Could you check a few things on this model? Use its own coordinates, in mm. Face numbers are marked on the shaded views. A direction names the side the tool comes from. Round coordinates to 2 decimals unless told otherwise and drop trailing zeros. Loops run counter-clockwise (first coordinate to the right, second up) from the corner with the lowest first, then second, coordinate; pieces in that order, holes last. Notation, with made-up numbers: M 23.25,83.25 L 36.25,83.25 A32 cw 36.25,117.25 Z; hole C 87,76.5 d6. An arc over 180 degrees is marked long. Answer in a Markdown table with one row per item.
```python
from build123d import *

# Parameters (mm, degrees)
F1_DEPTH         = 16
F2_T             = -2.5
F3_R             = 1
F4_DEPTH         = 5.5
F4_COPIES2_COUNT = 2
F5_W             = 11.5
F5_H             = 11.5
F5_R             = 2.75
F6_DEPTH         = 2.501


# Not quite as in the source:
# - a pattern or mirror of a feature is missing from the dataset's text; its kind, count and spacing are read off the source's solid


with BuildPart() as f1:
    # F0 (on Top) → F1 (new body)
    with BuildSketch(Plane.XY):
        with BuildLine():
            ThreePointArc((36.12, 24.13), (33.9115851301, 29.4615851301), (28.58, 31.67))
            Line((28.58, 31.67), (-28.58, 31.67))
            ThreePointArc((-28.58, 31.67), (-33.9115851301, 29.4615851301), (-36.12, 24.13))
            Line((-36.12, 24.13), (-36.12, -24.13))
            ThreePointArc((-36.12, -24.13), (-33.9115851301, -29.4615851301), (-28.58, -31.67))
            Line((-28.58, -31.67), (28.58, -31.67))
            ThreePointArc((28.58, -31.67), (33.9115851301, -29.4615851301), (36.12, -24.13))
            Line((36.12, -24.13), (36.12, 24.13))
        make_face()
    extrude(amount=F1_DEPTH)

    # F2
    f2_openings = [f1.faces().sort_by_distance(p)[0] for p in [
        (0, 0, 16),
    ]]
    offset(amount=F2_T, openings=f2_openings)

    # F3 (on face) → F4 (join)
    with BuildSketch(Plane.XY.offset(2.5)):
        with BuildLine():
            Line((-26.04, 24.13), (-26.04, 29.17))
            Line((-26.04, 29.17), (-28.58, 29.17))
            ThreePointArc((-28.58, 29.17), (-32.1438181772, 27.6938181772), (-33.62, 24.13))
            Line((-33.62, 24.13), (-33.62, 21.59))
            Line((-33.62, 21.59), (-28.58, 21.59))
            ThreePointArc((-28.58, 21.59), (-26.7839487758, 22.3339487758), (-26.04, 24.13))
        make_face()
        with Locations((-28.58, 24.13)):
            Circle(F3_R, mode=Mode.SUBTRACT)
    f4 = extrude(amount=F4_DEPTH)

    # F4_copies: F4 across plane
    add(f4.mirror(Plane(origin=(0, 0, 0), x_dir=(0, 0, 1), z_dir=(1, 0, 0))))

    # F4_copies1: F4 across plane
    add(f4.mirror(Plane(origin=(0, 0, 0), x_dir=(0, 0, -1), z_dir=(0, -1, 0))))

    # F4_copies2: F4 ×2 about axis
    f4_copies2_axis = Axis((0, 0, 0), (0, 0, 1))
    for i in range(1, F4_COPIES2_COUNT):
        add(f4.rotate(f4_copies2_axis, i * 360 / F4_COPIES2_COUNT))

    # F5 (on face) → F6 (cut, through all)
    with BuildSketch(Plane.XY.offset(2.5)):
        with Locations((-18.42, 13.97)):
            Rectangle(F5_W, F5_H)
        with Locations((-5.72, 13.97)):
            Circle(F5_R)
        with Locations((-18.42, -6.35)):
            Rectangle(F5_W, F5_H)
        with Locations((-5.72, -6.35)):
            Circle(F5_R)
        with Locations((13.33, 13.97)):
            Rectangle(F5_W, F5_H)
        with Locations((26.03, 13.97)):
            Circle(F5_R)
        with Locations((13.33, -6.35)):
            Rectangle(F5_W, F5_H)
        with Locations((26.03, -6.35)):
            Circle(F5_R)
    extrude(amount=-F6_DEPTH, mode=Mode.SUBTRACT)


solid = f1.part
```
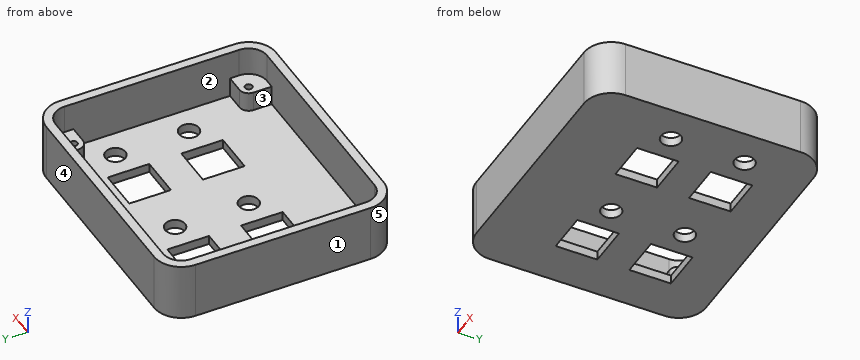
1) I want a section at C-C, the plane z = 5.5. Please give me the cut outline in (x, y).
Computed:
| item | result |
|---|---|
| outline | M -36.12,-24.13 A7.54 ccw -28.58,-31.67 L 28.58,-31.67 A7.54 ccw 36.12,-24.13 L 36.12,24.13 A7.54 ccw 28.58,31.67 L -28.58,31.67 A7.54 ccw -36.12,24.13 Z; hole M -33.62,-21.59 L -28.58,-21.59 A2.54 cw -26.04,-24.13 L -26.04,-29.17 L 26.04,-29.17 L 26.04,-24.13 A2.54 cw 28.58,-21.59 L 33.62,-21.59 L 33.62,21.59 L 28.58,21.59 A2.54 cw 26.04,24.13 L 26.04,29.17 L -26.04,29.17 L -26.04,24.13 A2.54 cw -28.58,21.59 L -33.62,21.59 Z; hole C -28.58,-24.13 d2; hole C -28.58,24.13 d2; hole C 28.58,-24.13 d2; hole C 28.58,24.13 d2 |
2) I want a section at D-D, the plane z = 10. Please give me the cut outline in (x, y), plus the area to 3 significant figures.
Computed:
| item | result |
|---|---|
| outline | M -36.12,-24.13 A7.54 ccw -28.58,-31.67 L 28.58,-31.67 A7.54 ccw 36.12,-24.13 L 36.12,24.13 A7.54 ccw 28.58,31.67 L -28.58,31.67 A7.54 ccw -36.12,24.13 Z; hole M -33.62,-24.13 A5.04 ccw -28.58,-29.17 L 28.58,-29.17 A5.04 ccw 33.62,-24.13 L 33.62,24.13 A5.04 ccw 28.58,29.17 L -28.58,29.17 A5.04 ccw -33.62,24.13 Z |
| area | 626 mm² |
3) I need wall thicknesses on line 1 (Y direction, x = 28.58, z = 5.25); line 2 (Y direction, x = -19, z = 5.25); line 3 (Y direction, x = 23.5, z = 1). Which ranges of each line are inside material? Lowest first, please.
Computed:
| item | result |
|---|---|
| line 1 | y = -31.67 to -25.13, -23.13 to -21.59, 21.59 to 23.13, 25.13 to 31.67 |
| line 2 | y = -31.67 to -29.17, 29.17 to 31.67 |
| line 3 | y = -31.67 to -7.43, -5.27 to 12.89, 15.05 to 31.67 |
4) I want a section at B-B, the plane y = -6.35. Please give me the cut outline in (x, z), plus the area to 3 significant figures.
Computed:
| item | result |
|---|---|
| outline | M -36.12,0 L -24.17,0 L -24.17,2.5 L -33.62,2.5 L -33.62,16 L -36.12,16 Z; M -12.67,0 L -8.47,0 L -8.47,2.5 L -12.67,2.5 Z; M -2.97,0 L 7.58,0 L 7.58,2.5 L -2.97,2.5 Z; M 19.08,0 L 23.28,0 L 23.28,2.5 L 19.08,2.5 Z; M 28.78,0 L 36.12,0 L 36.12,16 L 33.62,16 L 33.62,2.5 L 28.78,2.5 Z |
| area | 163 mm² |
5) Will these pins go through, and if not, where does the flat tip stop? P1, Ø2.5, axis at x = -28, y = -25, coming from the +Z side; P2, Ø1.5, axis at x = 30, z = 4.5, coming from the -Y side; P3, Ø10, axis at x = -4, y = -14.5, coming from the +Z side.
Computed:
| item | result |
|---|---|
| P1 | stops at z = 8 |
| P2 | stops at y = -31.64 |
| P3 | stops at z = 2.5 |
6) If we mould it in two halves opening along X, with no side actions, what happens to the marked faces 3, 4 and 5? For each: released by +X, released by -X, zero draft, split by the parting line, or undercut.
Computed:
| item | result |
|---|---|
| face 3 | undercut |
| face 4 | zero draft |
| face 5 | released by -X |
7) I want a section at A-A, the plane x = 11.5. Please give me the cut outline in (y, z).
Computed:
| item | result |
|---|---|
| outline | M -31.67,0 L -12.1,0 L -12.1,2.5 L -29.17,2.5 L -29.17,16 L -31.67,16 Z; M -0.6,0 L 8.22,0 L 8.22,2.5 L -0.6,2.5 Z; M 19.72,0 L 31.67,0 L 31.67,16 L 29.17,16 L 29.17,2.5 L 19.72,2.5 Z |
8) Which directions (+Z, -Z, +X, -X, +Y, -Y) give clear straight access to the entire face, cutting with the end or side of a thin tool? Please do the marked faces 1 and 2.
Computed:
| item | result |
|---|---|
| face 1 | +Z, -Z, -X, +Y, -Y |
| face 2 | +Z |
